from build123d import *

# Parameters (mm, degrees)
F1_DEPTH = 10
F2_W     = 24
F2_H     = 60
F3_DEPTH = 25
F4_R     = 5.556235
F4_R_2   = 5.60079
F4_R_3   = 5.912316
F5_DEPTH = 25


with BuildPart() as f1:
    # F0 (on Top) → F1 (new body)
    with BuildSketch(Plane.XY):
        Polygon((0, 52.050263), (-20, 33.911906), (-20, -36.088094), (20, -36.088094), (20, 33.911906), align=None)
    extrude(amount=F1_DEPTH)

    # F2 (on face) → F3 (join)
    with BuildSketch(Plane.XY.offset(10)):
        with Locations((0, 1.911906)):
            Rectangle(F2_W, F2_H)
    extrude(amount=F3_DEPTH)

    # F4 (on face) → F5 (join)
    with BuildSketch(Plane.XY.offset(35)):
        with Locations((0, 16.571494)):
            Circle(F4_R)
        Circle(F4_R_2)
        with Locations((0, -16.513106)):
            Circle(F4_R_3)
    extrude(amount=F5_DEPTH)


solid = f1.part
Geometry: final body of the model. Coordinates: model frame, mm. A direction names the side the tool comes from. Give positions to 0.01 mm unless a question says otherwise; leave off trailing zeros. Write each loop counter-clockwise with the first axis right and the second up, starting at its lowest first coordinate (ties: lowest second). Pieces come first, ordered by that corner, then holes. Notation, with made-up numbers: (-8, -24) -> (23, -24) arc R21 cw to (23, 12) -> close; hole circle Ø7 at (41, 32.5). An arc over 180 degrees is marked (long way). Answer as a JSON object with one key per item and string values.
1. Cut plane C-C on x = 10. Output: boundary loops of the cut face in (y, z), and give its area (3 significant figures).
Ans:
{"outline": "(-36.09, 0) -> (42.98, 0) -> (42.98, 10) -> (31.91, 10) -> (31.91, 35) -> (-28.09, 35) -> (-28.09, 10) -> (-36.09, 10) -> close", "area": "2,290 mm^2"}
2. Cut plane A-A on y = 7. Output: boundary loops of the cut face in (x, z), and give its area (3 significant figures).
Ans:
{"outline": "(-20, 0) -> (20, 0) -> (20, 10) -> (12, 10) -> (12, 35) -> (-12, 35) -> (-12, 10) -> (-20, 10) -> close", "area": "1,000 mm^2"}
3. Cut plane B-B on z = 5. Output: boundary loops of the cut face in (x, y), and give its area (3 significant figures).
Ans:
{"outline": "(-20, -36.09) -> (20, -36.09) -> (20, 33.91) -> (0, 52.05) -> (-20, 33.91) -> close", "area": "3,160 mm^2"}
4. Cut plane D-D on x = 3. Output: boundary loops of the cut face in (y, z).
Ans:
{"outline": "(-36.09, 0) -> (49.33, 0) -> (49.33, 10) -> (31.91, 10) -> (31.91, 35) -> (21.25, 35) -> (21.25, 60) -> (11.89, 60) -> (11.89, 35) -> (4.73, 35) -> (4.73, 60) -> (-4.73, 60) -> (-4.73, 35) -> (-11.42, 35) -> (-11.42, 60) -> (-21.61, 60) -> (-21.61, 35) -> (-28.09, 35) -> (-28.09, 10) -> (-36.09, 10) -> close"}
5. Ray query, probe 1 along Y at (x, z) = (1.5, 36); probe 2 along Y at (x, z) = (1, 54.5); probe 3 along Z at (x, y) = (16, 37). Return the intervals inside material, ascending. Write a range as from..to.
Ans:
{"probe 1": "y = -22.23..-10.79, -5.4..5.4, 11.22..21.92", "probe 2": "y = -22.34..-10.69, -5.51..5.51, 11.11..22.04", "probe 3": "z = 0..10"}
6. Mould query, pull axis Y, two halves, no side actions, for faces 6 (the flat face through (0, 9, 0)), 7 (the flat face through (10.14, 42.854, 4.93)), 8 (the flat face through (-6, 2, 35)), 9 (the cylindrical face through (-4.445, -3.408, 47.325)). Classes: pulls with the +Y half, pulls with the -Y half, needs draft (parallel to the pull), parting line crosses it, or undercut.
Ans:
{"face 6": "needs draft", "face 7": "pulls with the +Y half", "face 8": "undercut", "face 9": "undercut"}
7. Contact query for flat-ended pins moving along their axis: pin 1 (12 mm diameter, centred on x = -9, z = 20.5, fed in from +Y); pin 2 (6 mm diameter, centred on y = -17.5, z = 28.5, fed in from -X); pin 3 (7.5 mm diameter, centred on y = 10, z = 27, fed in from +X); pin 4 (12 mm diameter, centred on x = 13, z = 52, fed in from +Y). Output: stop coordinate, or through.
Ans:
{"pin 1": "stops at y = 31.91", "pin 2": "stops at x = -12", "pin 3": "stops at x = 12", "pin 4": "passes through"}
8. Access query for faces 1 (the flat face through (0, -28.088, 22)), 2 (the flat face through (12, 1, 22)), 3 (the cylindrical face through (-1.204, 11.147, 47.325)), 4 (the flat face through (0, 31.912, 22)), 5 (the flat face through (-12, 1, 22)). Directions: +Z, -Z, +X, -X, +Y, -Y. A direction counts if a zero-diameter tool reaches every point of the face in a straight line with its end or side. Return the directions, or none.
Ans:
{"face 1": "+Z, +X, -X, -Y", "face 2": "+Z, +X, +Y, -Y", "face 3": "+Z", "face 4": "+Z, +X, -X, +Y", "face 5": "+Z, -X, +Y, -Y"}
